```python
from build123d import *

# Parameters (mm, degrees)
SKETCH2_R      = 69.85
EXTRUDE1_DEPTH = 101.6


with BuildPart() as part:
    # Sketch2 → Extrude1 (new body)
    with BuildSketch(Plane(origin=(0, 0, 0), x_dir=(1, 0, 0), z_dir=(0, 1, 0))):
        Circle(SKETCH2_R)
    extrude(amount=EXTRUDE1_DEPTH)

    # Sketch5 → Revolve1 (revolve)
    with BuildSketch(Plane.XY):
        with BuildLine():
            Line((0, 171.45), (0, 101.6))
            Line((0, 101.6), (-69.85, 101.6))
            ThreePointArc((-69.85, 101.6), (-49.391408666, 150.991408666), (0, 171.45))
        make_face()
    revolve(axis=Axis((0, 101.6, 0), (0, -1, 0)))

    # Sketch6 → Revolve2 (revolve)
    with BuildSketch(Plane.XY):
        with BuildLine():
            Line((0, -69.85), (0, 0))
            Line((0, 0), (-69.85, 0))
            ThreePointArc((-69.85, 0), (-49.391408666, -49.391408666), (0, -69.85))
        make_face()
    revolve(axis=Axis((0, 0, 0), (0, 1, 0)))


solid = part.part
```
For this review, take the finished solid that the model builds, in its own axes (mm). Round coordinates to 2 decimals unless told otherwise and drop trailing zeros. Write each loop counter-clockwise with the first axis right and the second up, starting at its lowest first coordinate (ties: lowest second). Pieces come first, ordered by that corner, then holes. Notation, with made-up numbers: M -30.5,7.5 L 16.5,7.5 A30 cw 16.5,34.5 Z; hole C -9,2.5 d6. An arc over 180 degrees is marked long. One line per item, written item: value. Start each with the question number.
(1) We need section C-C (y = 76). Give the boundary of the cut face in (x, z), and give its area (3 significant figures).
(2) Wall thickness on line 1 (X direction, y = 151, z = -27.5); line 2 (X direction, y = -13.5, z = -8.5); line 3 (Z direction, x = 39.5, y = -27): over which ranges is each line inside the solid? List them lowest first.
(3) We need section D-D (y = 121). Give the boundary of the cut face in (x, z).
(4) We need section B-B (x = 0). Give the boundary of the cut face in (y, z).
(5) We need section A-A (z = 0). Give the boundary of the cut face in (x, y).
(6) Insertion check: pin 1 (1 mm diameter, centred on x = -4, z = -40.5, fed in from +Y); pin 2 (10 mm diameter, centred on x = -29.5, y = 106, fed in from -Z); pin 3 (5 mm diameter, centred on y = 43.5, z = -31, fed in from -X). Each pin has a flat end and moves straight along its axis. Give the tip position at first contact, or say it passes through.
Result:
1. outline: C 0,0 d139.7
1. area: 15,300 mm²
2. line 1: -41.02 to 41.02
2. line 2: -68 to 68
2. line 3: -50.89 to 50.89
3. outline: C 0,0 d134.2
4. outline: M 0,-69.85 L 101.6,-69.85 A69.85 ccw 101.6,69.85 L 0,69.85 A69.85 ccw Z
5. outline: M -69.85,0 A69.85 ccw 69.85,0 L 69.85,101.6 A69.85 ccw -69.85,101.6 Z
6. pin 1: y = 158.72
6. pin 2: z = -65.29
6. pin 3: x = -63.77
